Design review of the part built by this model. Coordinates are the model's own, in mm. Face numbers are marked on the shaded views. Coordinates: 2 decimals unless noted, no trailing zeros. Order: outer loops, then holes, each group sorted by start corner. A loop starts at its lowest first (then second) coordinate and runs counter-clockwise, first axis right, second up. Notation, with made-up numbers: (29, 77) -> (86, 77) arc R18 cw to (86, 86) -> close; hole circle Ø5 at (-37, 76.25). An arc over 180 degrees is marked (long way). Use a Markdown table: item, result. Add a question column.
Q1. Add section D-D (x = 1). Count the separate pieces of the cut face and the enclosed holes in it, then the cut area to 4 significant figures.
Q2. The part is to be moulded in two halves that separate along Y. For the marked faces 1, 2 and 3, say which applies: pulls with the +Y half, pulls with the -Y half, needs draft (parallel to the pull), parting line crosses it, or undercut.
Q3. Add section C-C (x = 15). State the section outline as (y, z) points.
Q4. Add section A-A (z = 5). State the section outline as (x, y) points (3 decimals), then the cut area to 3 significant figures.
Q5. Add section B-B (y = -26). State the section outline as (x, z) points, then the cut area to 3 significant figures.
Q6. Wall thickness on probe 1 along Y at (x, z) = (24.5, 4.5) (3 decimals); probe 2 along X at (y, z) = (-8.5, 2.75); probe 3 along Z at (x, y) = (9, -11.5): over which ranges is each line inside the solid? List them lowest first.
Q7. Insertion check: pin 1 (4 mm diameter, centred on x = 2.5, y = 9, fed in from +Z); pin 2 (3 mm diameter, centred on x = -1.5, z = 2.5, fed in from -Y); pin 3 (1.9 mm diameter, centred on x = -27, z = 5.5, fed in from +Y); pin 4 (3 mm diameter, centred on y = 14, z = -0.5, fed in from -X). Each pin has a flat end and moves straight along its axis. Give the tip position at first contact, or say it passes through.
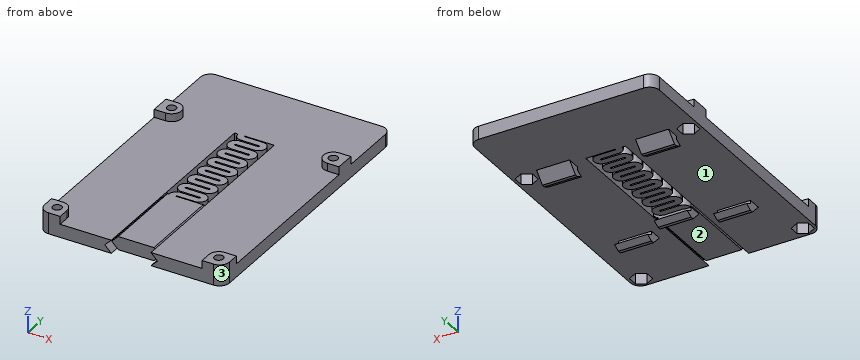
from build123d import *

# Parameters (mm, degrees)
PAD_DEPTH           = 4
PAD001_DEPTH        = 2.4
POCKET002_DEPTH     = 4
SKETCH006_R         = 1.375
POCKET003_DEPTH     = 206.380999
POCKET001_DEPTH     = 28.1
SKETCH007_W         = 12
SKETCH007_H         = 35
POCKET_DEPTH        = 6.401
PAD002_DEPTH        = 4
LINEARPATTERN_COUNT = 7
LINEARPATTERN_PITCH = 5
PAD003_DEPTH        = 25
PAD004_DEPTH        = 10
PAD005_DEPTH        = 10


with BuildPart() as part:
    # Sketch → Pad (new body)
    with BuildSketch(Plane.XY):
        with BuildLine():
            ThreePointArc((-25, 42.5), (-27.12132, 41.62132), (-28, 39.5))
            Line((-28, -39.5), (-28, 39.5))
            ThreePointArc((-28, -39.5), (-27.12132, -41.62132), (-25, -42.5))
            Line((25, -42.5), (-25, -42.5))
            ThreePointArc((25, -42.5), (27.12132, -41.62132), (28, -39.5))
            Line((28, 39.5), (28, -39.5))
            ThreePointArc((28, 39.5), (27.12132, 41.62132), (25, 42.5))
            Line((-25, 42.5), (25, 42.5))
        make_face()
    extrude(amount=PAD_DEPTH)

    # Sketch001 → Pad001 (join)
    with BuildSketch(Plane.XY.offset(4)):
        with BuildLine():
            ThreePointArc((-28, -39.5), (-27.12132, -41.62132), (-25, -42.5))
            Line((-25, -42.5), (-21.5, -42.5))
            Line((-21.5, -42.5), (-21.5, -39))
            ThreePointArc((-21.5, -39), (-22.37868, -36.87868), (-24.5, -36))
            Line((-28, -36), (-24.5, -36))
            Line((-28, -39.5), (-28, -36))
        make_face()
        with BuildLine():
            ThreePointArc((-24.5, 16), (-21.5, 19), (-24.5, 22))
            Line((-24.5, 22), (-28, 22))
            Line((-28, 16), (-28, 22))
            Line((-24.5, 16), (-28, 16))
        make_face()
    pad001 = extrude(amount=PAD001_DEPTH)

    # Sketch005 → Pocket002 (cut)
    with BuildSketch(Plane.XY):
        Polygon((-21.901924, -40.5), (-21.901924, -37.5), (-24.5, -36), (-27.098076, -37.5), (-27.098076, -40.5), (-24.5, -42), align=None)
        Polygon((-21.901924, 17.5), (-21.901924, 20.5), (-24.5, 22), (-27.098076, 20.5), (-27.098076, 17.5), (-24.5, 16), align=None)
    pocket002 = extrude(amount=POCKET002_DEPTH, mode=Mode.SUBTRACT)

    # Sketch006 → Pocket003 (cut, through all)
    with BuildSketch(Plane.XY.offset(4)):
        with Locations((-24.5, 19)):
            Circle(SKETCH006_R)
        with Locations((-24.5, -39)):
            Circle(SKETCH006_R)
    pocket003 = extrude(amount=POCKET003_DEPTH, mode=Mode.SUBTRACT)

    # Sketch003 → Pocket001 (cut)
    with BuildSketch(Plane.XZ.offset(42.5)):
        Polygon((-6, 0), (-8, 2), (-6, 4), (6, 4), (8, 2), (6, 0), align=None)
    extrude(amount=-POCKET001_DEPTH, mode=Mode.SUBTRACT)

    # Sketch007 → Pocket (cut, through all)
    with BuildSketch(Plane.XY):
        with Locations((0, 2.5)):
            Rectangle(SKETCH007_W, SKETCH007_H)
    extrude(amount=POCKET_DEPTH, mode=Mode.SUBTRACT)

    # Sketch009 → Pad002 (join)
    with BuildSketch(Plane.XY):
        with BuildLine():
            Line((-5, 20), (-3, 20))
            ThreePointArc((-3, 20), (-2.926777, 19.823223), (-2.75, 19.75))
            Line((-2.75, 19.75), (2.75, 19.75))
            ThreePointArc((2.75, 15.25), (5, 17.5), (2.75, 19.75))
            Line((2.75, 15.25), (-2.75, 15.25))
            ThreePointArc((-2.75, 15.25), (-2.926777, 15.176777), (-3, 15))
            Line((-5, 15), (-3, 15))
            ThreePointArc((-2.75, 17.25), (-4.34099, 16.59099), (-5, 15))
            Line((2.75, 17.25), (-2.75, 17.25))
            ThreePointArc((2.75, 17.25), (3, 17.5), (2.75, 17.75))
            Line((-2.75, 17.75), (2.75, 17.75))
            ThreePointArc((-5, 20), (-4.34099, 18.40901), (-2.75, 17.75))
        make_face()
    pad002 = extrude(amount=PAD002_DEPTH)

    # LinearPattern: Pad002 ×7
    with Locations(*[(0, -i * LINEARPATTERN_PITCH, 0) for i in range(1, LINEARPATTERN_COUNT)]):
        add(pad002)

    # Sketch008 → Pad003 (join)
    with BuildSketch(Plane.XZ.offset(15)):
        Polygon((-5.4, 0), (5.4, 0), (7.4, 2), (5.4, 4), (-5.4, 4), (-7.4, 2), align=None)
    extrude(amount=PAD003_DEPTH)

    # Sketch010 → Pad004 (join)
    with BuildSketch(Plane.YZ.offset(5)):
        Polygon((-19, 0), (-15, 0), (-15, -1), (-13, -2), (-15, -3), (-16, -3), align=None)
    extrude(amount=-PAD004_DEPTH)

    # Sketch011 → Pad005 (join)
    with BuildSketch(Plane.YZ.offset(10)):
        Polygon((-20, 0), (-20, -1), (-18, -2), (-20, -3), (-21, -3), (-24, 0), align=None)
        Polygon((17.5, 0), (17.5, -1), (15.5, -2), (17.5, -3), (18.5, -3), (21.5, 0), align=None)
    pad005 = extrude(amount=PAD005_DEPTH)

    # Mirrored: Pad001, Pocket002, Pocket003, Pad005 across Sketch001 V_Axis
    add(pad001.mirror(Plane(origin=(0, 0, 4), x_dir=(0, 0, 1), z_dir=(1, 0, 0))))
    add(pocket002.mirror(Plane(origin=(0, 0, 4), x_dir=(0, 0, 1), z_dir=(1, 0, 0))), mode=Mode.SUBTRACT)
    add(pocket003.mirror(Plane(origin=(0, 0, 4), x_dir=(0, 0, 1), z_dir=(1, 0, 0))), mode=Mode.SUBTRACT)
    add(pad005.mirror(Plane(origin=(0, 0, 4), x_dir=(0, 0, 1), z_dir=(1, 0, 0))))


solid = part.part
Established:
| question | item | result |
|---|---|---|
| 1 | separate pieces | 16 |
| 1 | enclosed holes | 0 |
| 1 | area | 311.5 mm^2 |
| 2 | face 1 | undercut |
| 2 | face 2 | needs draft |
| 2 | face 3 | pulls with the -Y half |
| 3 | outline | (-42.5, 0) -> (-24, 0) -> (-21, -3) -> (-20, -3) -> (-18, -2) -> (-20, -1) -> (-20, 0) -> (17.5, 0) -> (17.5, -1) -> (15.5, -2) -> (17.5, -3) -> (18.5, -3) -> (21.5, 0) -> (42.5, 0) -> (42.5, 4) -> (-42.5, 4) -> close |
| 4 | outline | (-28, -39.5) arc R3 ccw to (-25, -42.5) -> (-21.5, -42.5) -> (-21.5, -39) arc R3 ccw to (-24.5, -36) -> (-28, -36) -> close; (-28, 16) -> (-24.5, 16) arc R3 ccw to (-24.5, 22) -> (-28, 22) -> close; (21.5, -42.5) -> (25, -42.5) arc R3 ccw to (28, -39.5) -> (28, -36) -> (24.5, -36) arc R3 ccw to (21.5, -39) -> close; (24.5, 16) -> (28, 16) -> (28, 22) -> (24.5, 22) arc R3 ccw to start; hole circle Ø2.75 at (-24.5, -39); hole circle Ø2.75 at (-24.5, 19); hole circle Ø2.75 at (24.5, -39); hole circle Ø2.75 at (24.5, 19) |
| 4 | area | 123 mm^2 |
| 5 | outline | (-28, 0) -> (-6, 0) -> (-8, 2) -> (-6, 4) -> (-28, 4) -> close; (-7.4, 2) -> (-5.4, 0) -> (5.4, 0) -> (7.4, 2) -> (5.4, 4) -> (-5.4, 4) -> close; (6, 0) -> (28, 0) -> (28, 4) -> (6, 4) -> (8, 2) -> close |
| 5 | area | 219 mm^2 |
| 6 | probe 1 | -42.5 to -40.375, -37.625 to -36, 16 to 17.625, 20.375 to 22 |
| 6 | probe 2 | -28 to -6, -4.43 to 4.77, 6 to 28 |
| 6 | probe 3 | 0 to 4 |
| 7 | pin 1 | z = 4 |
| 7 | pin 2 | y = -40 |
| 7 | pin 3 | y = 22 |
| 7 | pin 4 | x = -28 |
